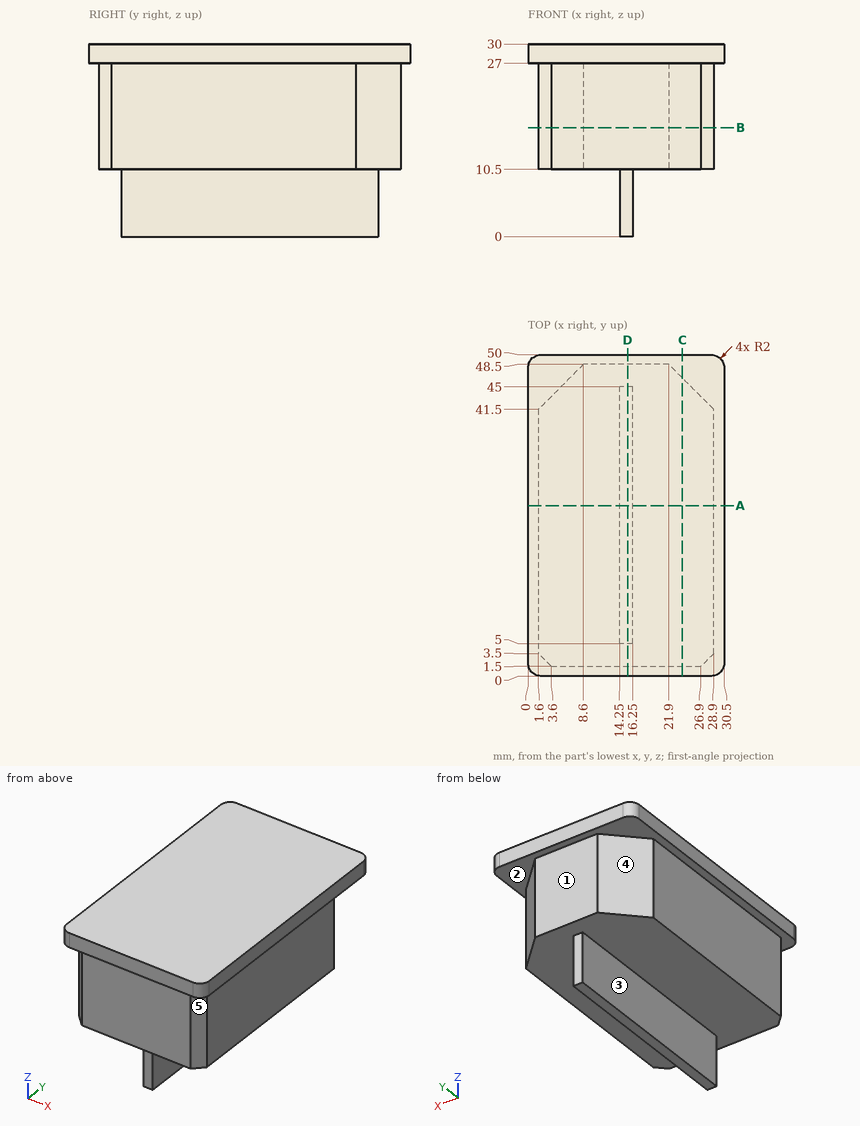
Verification items for this drawing (mm, ordinates from the low corner). A direction names the side the tool comes from. Round coordinates to 2 decimals unless told otherwise and drop trailing zeros. Order: outer loops, then holes, each group sorted by start corner. A loop starts at its lowest first (then second) coordinate and runs counter-clockwise, first axis right, second up. Notation, with made-up numbers: M 34,43 L 85,43 A15 ccw 85,62 Z; hole C 87.5,3 d3. An arc over 180 degrees is marked long. Answer in a Markdown table with one row per item. Add a question column.
Item 1: Depth check by flat-ended pin: pin 1 Ø10.5 at (x, z) = (13.5, 19.5) entering from +Y; pin 2 Ø6 at (y, z) = (11.5, 10) entering from -X; pin 3 Ø3 at (y, z) = (25.5, 19) entering from +X. Enter the tip coordinate at first touch or a pass-through.
Item 2: Sectioned sample at A-A, the plane y = 26.5. Enter the section's corners in (x, z).
Item 3: Set-up check for the marked faces 1, 2, 3, 4 and 5: record each of +Z, -Z, +X, -X, +Y, -Y from which the full face is reachable in a straight line by a thin tool's end or side.
Item 4: Sectioned sample at C-C, the plane x = 24. Enter the section's corners in (y, z), plus the area to 3 significant figures.
Item 5: Sectioned sample at D-D, the plane x = 15.5. Enter the section's corners in (y, z).
Item 6: Sectioned sample at B-B, the plane z = 17. Enter the section's corners in (x, y).
Item 7: Material ranges on L1, parallel to Y at x = 19.5, z = 14.25; L2, parallel to Z at x = 18, y = 42; L3, parallel to X at y = 37, z = 17.25, recorded low to high. Write a range as [from, to].
Filled in:
| question | item | result |
|---|---|---|
| 1 | pin 1 | stops at y = 48.5 |
| 1 | pin 2 | stops at x = 1.6 |
| 1 | pin 3 | stops at x = 28.9 |
| 2 | outline | M 0,27 L 1.6,27 L 1.6,10.5 L 14.25,10.5 L 14.25,0 L 16.25,0 L 16.25,10.5 L 28.9,10.5 L 28.9,27 L 30.5,27 L 30.5,30 L 0,30 Z |
| 3 | face 1 | -Z, +X, -X, +Y |
| 3 | face 2 | -Z |
| 3 | face 3 | -Z, -X, +Y, -Y |
| 3 | face 4 | -Z, -X, +Y |
| 3 | face 5 | -Z, +X, -Y |
| 4 | outline | M 0,27 L 1.5,27 L 1.5,10.5 L 46.4,10.5 L 46.4,27 L 50,27 L 50,30 L 0,30 Z |
| 4 | area | 891 mm² |
| 5 | outline | M 0,27 L 1.5,27 L 1.5,10.5 L 5,10.5 L 5,0 L 45,0 L 45,10.5 L 48.5,10.5 L 48.5,27 L 50,27 L 50,30 L 0,30 Z |
| 6 | outline | M 1.6,3.5 L 3.6,1.5 L 26.9,1.5 L 28.9,3.5 L 28.9,41.5 L 21.9,48.5 L 8.6,48.5 L 1.6,41.5 Z |
| 7 | L1 | y = [1.5, 48.5] |
| 7 | L2 | z = [10.5, 30] |
| 7 | L3 | x = [1.6, 28.9] |
